CAD build for the part. Positions are in the model's coordinates, mm. Coordinates: 2 decimals unless noted, no trailing zeros. Write item = value, one per line.
from build123d import *

# Parameters (mm, degrees)
F1_DEPTH       = 2.5
F2_D           = 3.5
F2_CSINK_D     = 6
F2_CSINK_ANGLE = 90
F3_T1_DEPTH    = 141.3928063628
F3_T4_ANGLE    = 86.5781008802
F3_T6_ANGLE    = 95.6855323437
F3_T8_ANGLE    = 105.4133416791
F3_T10_ANGLE   = 78.1582231343
F4_D           = 11.8
F5_D           = 8
F6_D           = 9


# Not quite as in the source:
# - a fillet or chamfer that OpenCascade refuses, or shapes differently, is made with other operations: its cross-section is extruded or revolved along the edge and cut away or added


with BuildPart() as f1:
    # F0 (on Front) → F1 (new body)
    with BuildSketch(Plane.XZ):
        with BuildLine():
            ThreePointArc((51.9193532242, 6.9790848915), (29.3726830737, 52.5798387856), (-17.6447437911, 72))
            ThreePointArc((-17.6447437911, 72), (-70.6003478325, 54.2753932247), (-101.9138280482, 8.0377068475))
            ThreePointArc((-101.9138280482, 8.0377068475), (-100.843919646, 2.5025617927), (-95.7922150584, 0))
            Line((-95.7922150584, 0), (45.6005913044, 0))
            ThreePointArc((45.6005913044, 0), (50.3078829387, 2.0880866422), (51.9193532242, 6.9790848915))
        make_face()
    extrude(amount=-F1_DEPTH)

    # F2 (through all)
    with Locations(Plane.XZ):
        with Locations((-92.7765071392, 19.3704143167), (-28.6957714707, 67.0258700848), (45.8813235164, 13.6932386085), (-41.5233448148, 4.6045258641)):
            CounterSinkHole(F2_D / 2, F2_CSINK_D / 2, counter_sink_angle=F2_CSINK_ANGLE)

    # F3: chamfer of 2 on 1 edges, made by hand

    # F3_s2 → F3_t1 (cut)
    with BuildSketch(Plane.YZ.offset(-95.7922150584)):
        Polygon((0, 2), (2, 0), (0, 0), align=None)
    extrude(amount=F3_T1_DEPTH, mode=Mode.SUBTRACT)

    # F3_s3 → F3_t4 (revolve, cut)
    with BuildSketch(Plane(origin=(-0.1784402108, 0, 1.7923196444), x_dir=(0, 1, 0), z_dir=(0.0990684869, 0, -0.9950806173))):
        Polygon((2, 52.3553494356), (0, 50.3553494356), (0, 52.3553494356), align=None)
    revolve(axis=Axis((-19.9365535802, 0, -0.1747635854), (0, -1, 0)), revolution_arc=F3_T4_ANGLE, mode=Mode.SUBTRACT)

    # F3_s5 → F3_t6 (revolve, cut)
    with BuildSketch(Plane.YZ.offset(45.6005913044)):
        Polygon((2, 0), (0, 2), (0, 0), align=None)
    revolve(axis=Axis((45.6005913044, 0, 6.35), (0, -1, 0)), revolution_arc=F3_T6_ANGLE, mode=Mode.SUBTRACT)

    # F3_s7 → F3_t8 (revolve, cut)
    with BuildSketch(Plane(origin=(-5.1396919269, 0, -18.6425770032), x_dir=(0, 1, 0), z_dir=(0.2657806059, 0, 0.9640335417))):
        Polygon((0, 98.3846151976), (2, 100.3846151976), (0, 100.3846151976), align=None)
    revolve(axis=Axis((-95.7922150584, 0, 6.35), (0, -1, 0)), revolution_arc=F3_T8_ANGLE, mode=Mode.SUBTRACT)

    # F3_s9 → F3_t10 (revolve, cut)
    with BuildSketch(Plane(origin=(-16.9209977533, 0, 1.0561482837), x_dir=(0, 1, 0), z_dir=(0.9980577677, 0, -0.0622952035))):
        Polygon((2, 70.9128484948), (0, 68.9128484948), (0, 70.9128484948), align=None)
    revolve(axis=Axis((-17.9304192048, 0, -15.1162191548), (0, -1, 0)), revolution_arc=F3_T10_ANGLE, mode=Mode.SUBTRACT)

    # F4 (through all)
    with Locations(Plane.XZ):
        with Locations((-61.7667548358, 20.886823535)):
            Hole(F4_D / 2)

    # F5 (through all)
    with Locations(Plane.XZ):
        with Locations((-19.6185931563, 20.886823535), (22.0020785928, 20.886823535)):
            Hole(F5_D / 2)

    # F6 (through all)
    with Locations(Plane.XZ):
        with Locations((-17.6447437911, 50.9389452636)):
            Hole(F6_D / 2)


solid = f1.part
(1) Wall check: line 1 (Z direction, x = 23.5, y = 1.5); line 2 (Z direction, x = -93.5, y = 2.3); line 3 (X direction, y = 2.05, z = 10). Give the ranges that are in metal, low to high. Write a range as from..to.
Evaluation:
line_1 = 0.5..17.18, 24.6..56.88
line_2 = 0..17.78, 20.96..28.23
line_3 = -101.35..51.55
(2) Pull direction X, two halves, no side cores. Call faces 1 (the face through (-26, 0, 29)), 2 (the face through (-100.893, 2.246, 2.568)), 3 (the face through (-67.22, 1.27, 18.63)), 4 (the face through (-19.098, 1.268, 24.853)): +X half, -X half, draft (parallel to the pull), parting line (faces both ways), or undercut.
Evaluation:
face_1 = draft
face_2 = -X half
face_3 = undercut
face_4 = undercut
(3) Slice it at A-A, the plane y = 0.7. State how many separate pieces and enclosed holes the cut face has, then the cut area to 3 significant figures.
Evaluation:
separate_pieces = 1
enclosed_holes = 8
area = 7,730 mm²
(4) Pin check, flat tip, straight feed: pin 1 Ø3 at (x, z) = (-28.7, 67.03) entering from +Y. Stop position of the tip, or through.
Evaluation:
pin_1 = through
